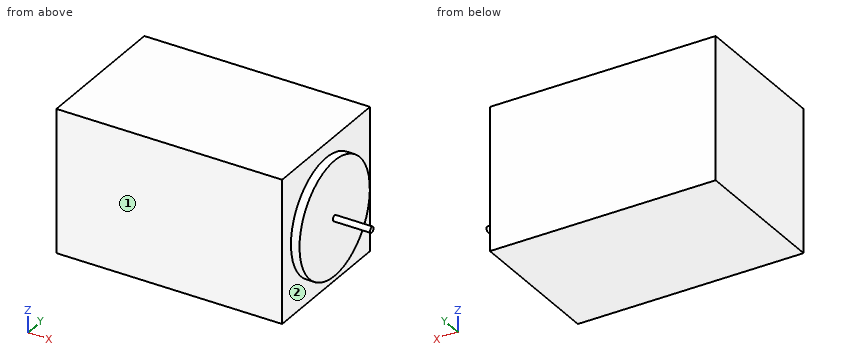
from build123d import *

# Parameters (mm, degrees)
SKETCH_1_W      = 50
SKETCH_1_H      = 50
EXTRUDE_1_DEPTH = 79
SKETCH_2_R      = 20
EXTRUDE_2_DEPTH = 82
SKETCH_3_R      = 1
EXTRUDE_3_DEPTH = 95


with BuildPart() as part:
    # 草图1 → 凸台-拉伸1 (new body)
    with BuildSketch(Plane(origin=(0, 0, 0), x_dir=(0, 0, -1), z_dir=(1, 0, 0))):
        Rectangle(SKETCH_1_W, SKETCH_1_H)
    extrude(amount=EXTRUDE_1_DEPTH)

    # 草图2 → 凸台-拉伸2 (add)
    with BuildSketch(Plane(origin=(0, 0, 0), x_dir=(0, 0, -1), z_dir=(1, 0, 0))):
        Circle(SKETCH_2_R)
    extrude(amount=EXTRUDE_2_DEPTH)

    # 草图3 → 凸台-拉伸3 (add)
    with BuildSketch(Plane(origin=(0, 0, 0), x_dir=(0, 0, -1), z_dir=(1, 0, 0))):
        Circle(SKETCH_3_R)
    extrude(amount=EXTRUDE_3_DEPTH)


solid = part.part
CAD build for the part. Positions are in the model's coordinates, mm. Face numbers are marked on the shaded views. A direction names the side the tool comes from. Give positions to 0.01 mm unless a question says otherwise; leave off trailing zeros. Order: outer loops, then holes, each group sorted by start corner. A loop starts at its lowest first (then second) coordinate and runs counter-clockwise, first axis right, second up. Notation, with made-up numbers: (8, 17) - (43, 17) arc R25 cw to (43, 52) - close; hole circle Ø5 at (79, 83). An arc over 180 degrees is marked (long way). Write each question's results on one line, items separated by ' | '.
1. Saw through at D-D on y = -5. List the corners of the cut face in (x, z), and give its area (3 significant figures).
Calculated:
outline: (0, -25) - (79, -25) - (79, -19.36) - (82, -19.36) - (82, 19.36) - (79, 19.36) - (79, 25) - (0, 25) - close | area: 4,070 mm2
2. Saw through at C-C on x = 83. List the corners of the cut face in (y, z), and give its area (3 significant figures).
Calculated:
outline: circle Ø2 at (0, 0) | area: 3.14 mm2
3. Saw through at A-A on y = 0. List the corners of the cut face in (x, z), and give its area (3 significant figures).
Calculated:
outline: (0, -25) - (79, -25) - (79, -20) - (82, -20) - (82, -1) - (95, -1) - (95, 1) - (82, 1) - (82, 20) - (79, 20) - (79, 25) - (0, 25) - close | area: 4,100 mm2
4. Pin check, flat tips, straight feed: pin 1 (2 mm diameter, centred on y = -11.5, z = 11.5, fed in from -X); pin 2 (10 mm diameter, centred on y = -14, z = 12, fed in from +X). Stop position of each tip, or through.
Calculated:
pin 1: stops at x = 0 | pin 2: stops at x = 82
5. Probe L1, parallel to X at y = 3, z = 9; L2, parallel to X at y = 4.5, z = -21; L3, parallel to Z at x = 81.5, y = -2.5. List the from-to ranges inside material, lowest first. Write a range as from..to.
Calculated:
L1: x = 0..82 | L2: x = 0..79 | L3: z = -19.84..19.84
6. 3-axis set-ups, long thin cutter, end or side, ignore diameter. For the marked faces 1 and 2: which of +Z, -Z, +X, -X, +Y, -Y reach the whole face in a straight line?
Calculated:
face 1: +Z, -Z, +X, -X, -Y | face 2: +X
